from build123d import *

# Parameters (mm, degrees)
CROQUIS1_W              = 70
CROQUIS1_H              = 55
SALIENTE_EXTRUIR1_DEPTH = 70
CROQUIS2_R              = 9.525
SALIENTE_EXTRUIR2_DEPTH = 10
CROQUIS3_R              = 9.525
REDONDEO1_R             = 4
CROQUIS5_W              = 42.976896334
CROQUIS5_H              = 90.412198776
CORTAR_EXTRUIR2_DEPTH   = 70


with BuildPart() as part:
    # Croquis1 → Saliente-Extruir1 (new body)
    with BuildSketch(Plane.XY):
        with Locations((35, -27.5)):
            Rectangle(CROQUIS1_W, CROQUIS1_H)
    extrude(amount=SALIENTE_EXTRUIR1_DEPTH)

    # Croquis2 → Saliente-Extruir2 (add)
    with BuildSketch(Plane.XZ.offset(55)):
        with Locations(Location((35, 35, 0), (0, 0, 90))):
            Circle(CROQUIS2_R)
    extrude(amount=SALIENTE_EXTRUIR2_DEPTH)

    # Barrer1: sweep along a curve in space
    with BuildLine() as barrer1_path:
        Line((35, -65, 35), (35, -854, 35))
        ThreePointArc((35, -854, 35), (31.778174593, -861.778174593, 35), (24, -865, 35))
        Line((24, -865, 35), (-14, -865, 35))
        ThreePointArc((-14, -865, 35), (-21.778174593, -861.778174593, 35), (-25, -854, 35))
        Line((-25, -854, 35), (-25, -805, 35))
    # Croquis3 → Barrer1 (sweep)
    with BuildSketch(Plane.XZ.offset(65)):
        with Locations((35, 35)):
            Circle(CROQUIS3_R)
    sweep(path=barrer1_path.line)

    # Redondeo1
    redondeo1_edges = [part.edges().sort_by_distance(p)[0] for p in [
        (-15.475, -805, 35),
    ]]
    fillet(redondeo1_edges, radius=REDONDEO1_R)

    # Croquis5 → Cortar-Extruir2 (cut)
    with BuildSketch(Plane.XY):
        with Locations((5.153209537, -811.315289476)):
            Rectangle(CROQUIS5_W, CROQUIS5_H)
    extrude(amount=CORTAR_EXTRUIR2_DEPTH, mode=Mode.SUBTRACT)


solid = part.part
Source: CAD feature listing. Evaluate the final solid. Frame: model axes, mm. A direction names the side the tool comes from. Round coordinates to 2 decimals unless told otherwise and drop trailing zeros. Loops run counter-clockwise (first coordinate to the right, second up) from the corner with the lowest first, then second, coordinate; pieces in that order, holes last.
Q1. Mould query, pull axis Y, two halves, no side actions, for faces 1 (the face through (43.841, -460.093, 38.545)), 2 (the face through (35, 0, 35)), 3 (the face through (35, -27, 0)). Classes: pulls with the +Y half, pulls with the -Y half, needs draft (parallel to the pull), parting line crosses it, or undercut.
Q2. Section B-B, the plane x = 61. Return loops of the section in (y, z), plus the area to 3 significant figures.
Q3. Ray query, line 1 (X direction, y = -823.5, z = 36); line 2 (Y direction, x = 60.5, z = 48); line 3 (X direction, y = -371.5, z = 36). Return the intervals inside material, ascending.
Q4. Section A-A, the plane z = 58.5. Return loops of the section in (x, y).
Q5. Access query for faces 4 (the face through (42, -55, 42)), 5 (the face through (-34.52, -831.18, 34.64)), 6 (the face through (0, -28, 35)), 7 (the face through (35, -27, 70)), 8 (the face through (70, -28, 35)). Directions: +Z, -Z, +X, -X, +Y, -Y. A direction counts if a zero-diameter tool reaches every point of the face in a straight line with its end or side. Return the directions, or none.
Q6. First-contact query: P1, Ø3, axis at x = 50, z = 19.5, coming from the -Y side; P2, Ø13.5, axis at y = -795, z = 35, coming from the -X side; P3, Ø8, axis at x = 38.5, y = -374.5, coming from the +Z side (3 decimals). Flat tips, straight axial feed; report the tip coordinate or a pass-through.
Q7. Section C-C, the plane y = -108. Return loops of the section in (x, z) (3 decimals), plus the area to 3 significant figures.
Solutions:
1. face 1: undercut
1. face 2: pulls with the +Y half
1. face 3: needs draft
2. outline: (-55, 0) - (0, 0) - (0, 70) - (-55, 70) - close
2. area: 3,850 mm2
3. line 1: x = -34.47 to -16.34, 26.64 to 44.47
3. line 2: y = -55 to 0
3. line 3: x = 25.53 to 44.47
4. outline: (0, -55) - (70, -55) - (70, 0) - (0, 0) - close
5. face 4: none
5. face 5: +Y
5. face 6: +Z, -Z, -X, +Y
5. face 7: +Z, +X, -X, +Y, -Y
5. face 8: +Z, -Z, +X, +Y, -Y
6. P1: stops at y = -55
6. P2: stops at x = 26.64
6. P3: stops at z = 44.525
7. outline: circle Ø19.05 at (35, 35)
7. area: 285 mm2
